CAD build for the part. Positions are in the model's coordinates, mm. A direction names the side the tool comes from. Give positions to 0.01 mm unless a question says otherwise; leave off trailing zeros. Write each loop counter-clockwise with the first axis right and the second up, starting at its lowest first coordinate (ties: lowest second). Pieces come first, ordered by that corner, then holes. Notation, with made-up numbers: (-22, 12.5) - (4, 12.5) arc R22 cw to (4, 48.5) - close; hole circle Ø6 at (47.25, 80). An arc over 180 degrees is marked (long way). Put each result on its own line as item: value. Start each with the question number.
1. Cut at D-D on x = -7.5. List the corners of the cut face in (y, z).
2. Mould opens along X. For faces 1 (the cylindrical face through (16.24, -12.517, 0.76)), 2 (the flat face through (19.5, 0, 1)), 3 (the cylindrical face through (-16.76, 16.483, 0.76)), 4 (the flat face through (-19.5, 0, 1)) say: +X half, -X half, draft (parallel to the pull), parting line (faces both ways), or undercut.
3. Drop flat-ended pins along their axis: pin 1 (2.5 mm diameter, centred on x = -8, z = 7, fed in from +Y); pin 2 (1 mm diameter, centred on y = 0, z = 6, fed in from -X); pin 3 (2 mm diameter, centred on x = 14.5, y = 9.5, fed in from +Z); pin 4 (3.5 mm diameter, centred on x = 16.5, y = -14.5, fed in from -Z) (3 decimals). Give the stop position or say it passes through.
4. Tool access for faces 5 (the flat face through (16.5, 0, 5)), 6 (the flat face through (-3.454, 15, 6)), 7 (the flat face through (-12.5, 15, 6)), 8 (the flat face through (11.5, -14, 5)): list every direction of +Z, -Z, +X, -X, +Y, -Y with a clear straight run to the whole face (end or side of a thin tool).
5. Wall check: line 1 (Y direction, x = 16.5, z = 1.1); line 2 (Y direction, x = -10.5, z = 4.5); line 3 (Y direction, x = -1, z = 7.25). Give the ranges that are in metal, low to high.
6. Cut at B-B on y = -14.5. List the corners of the cut face in (x, z), and give its area (4 significant figures).
7. Cut at A-A on x = -16.5. List the corners of the cut face in (y, z).
8. Cut at C-C on z = 8.25. List the corners of the cut face in (x, y), and give its area (3 significant figures).
from build123d import *

# Parameters (mm, degrees)
ESQUISSE1_W                     = 39
ESQUISSE1_H                     = 35
BOSS_EXTRU_1_DEPTH              = 1.5
ENL_V_MAT_EXTRU_1_REACH         = 28.244
ESQUISSE2_R                     = 2
R_P_TITION_LIN_AIRE1_COUNT      = 2
R_P_TITION_LIN_AIRE1_PITCH      = 33
R_P_TITION_LIN_AIRE1_COUNT_DIR2 = 2
R_P_TITION_LIN_AIRE1_PITCH_DIR2 = 29
ESQUISSE3_W                     = 9.045882094
ESQUISSE3_H                     = 2
BOSS_EXTRU_2_DEPTH              = 9
BOSS_EXTRU_3_DEPTH              = 8


with BuildPart() as part:
    # Esquisse1 → Boss.-Extru.1 (new body)
    with BuildSketch(Plane.XY):
        Rectangle(ESQUISSE1_W, ESQUISSE1_H)
    extrude(amount=BOSS_EXTRU_1_DEPTH)

    # Esquisse2 → Enlèv. mat.-Extru.1 (cut, up to next)
    with BuildSketch(Plane.XY.offset(1.5), mode=Mode.PRIVATE) as enl_v_mat_extru_1_sk1:
        with Locations((16.5, 14.5)):
            Circle(ESQUISSE2_R)
    enl_v_mat_extru_1_tool1 = extrude(enl_v_mat_extru_1_sk1.sketch, amount=-ENL_V_MAT_EXTRU_1_REACH, mode=Mode.PRIVATE) & part.part
    enl_v_mat_extru_1 = enl_v_mat_extru_1_tool1.solids().sort_by_distance((16.5, 14.5, 1.5))[0]
    add(enl_v_mat_extru_1, mode=Mode.SUBTRACT)

    # Répétition linéaire1: Enl_v. mat.-Extru.1 2 × 2
    with Locations(*[(-i * R_P_TITION_LIN_AIRE1_PITCH, -j * R_P_TITION_LIN_AIRE1_PITCH_DIR2, 0) for i in range(R_P_TITION_LIN_AIRE1_COUNT) for j in range(R_P_TITION_LIN_AIRE1_COUNT_DIR2) if (i, j) != (0, 0)]):
        add(enl_v_mat_extru_1, mode=Mode.SUBTRACT)

    # Esquisse3 → Boss.-Extru.2 (add)
    with BuildSketch(Plane.XY.offset(1.5)):
        with Locations((-7.977058953, 15.5)):
            Rectangle(ESQUISSE3_W, ESQUISSE3_H)
    extrude(amount=BOSS_EXTRU_2_DEPTH)

    # Esquisse4 → Boss.-Extru.3 (add)
    with BuildSketch(Plane.XY.offset(1.5)):
        Polygon((-13.5, 10.5), (16.5, 10.5), (16.5, -11.5), (11.5, -11.5), (11.5, -16.5), (-13.5, -16.5), align=None)
    extrude(amount=BOSS_EXTRU_3_DEPTH)


solid = part.part
Report:
1. outline: (-17.5, 0) - (17.5, 0) - (17.5, 1.5) - (16.5, 1.5) - (16.5, 10.5) - (14.5, 10.5) - (14.5, 1.5) - (10.5, 1.5) - (10.5, 9.5) - (-16.5, 9.5) - (-16.5, 1.5) - (-17.5, 1.5) - close
2. face 1: undercut
2. face 2: +X half
2. face 3: undercut
2. face 4: -X half
3. pin 1: stops at y = 16.5
3. pin 2: stops at x = -13.5
3. pin 3: stops at z = 9.5
3. pin 4: passes through
4. face 5: +Z, +X, +Y, -Y
4. face 6: +Z, +X, +Y
4. face 7: +Z, -X, +Y
4. face 8: +Z, +X, -Y
5. line 1: y = -17.5 to -16.5, -12.5 to 12.5, 16.5 to 17.5
5. line 2: y = -16.5 to 10.5, 14.5 to 16.5
5. line 3: y = -16.5 to 10.5
6. outline: (-19.5, 0) - (-18.5, 0) - (-18.5, 1.5) - (-19.5, 1.5) - close; (-14.5, 0) - (14.5, 0) - (14.5, 1.5) - (11.5, 1.5) - (11.5, 9.5) - (-13.5, 9.5) - (-13.5, 1.5) - (-14.5, 1.5) - close; (18.5, 0) - (19.5, 0) - (19.5, 1.5) - (18.5, 1.5) - close
6. area: 246.5 mm²
7. outline: (-17.5, 0) - (-16.5, 0) - (-16.5, 1.5) - (-17.5, 1.5) - close; (-12.5, 0) - (12.5, 0) - (12.5, 1.5) - (-12.5, 1.5) - close; (16.5, 0) - (17.5, 0) - (17.5, 1.5) - (16.5, 1.5) - close
8. outline: (-13.5, -16.5) - (11.5, -16.5) - (11.5, -11.5) - (16.5, -11.5) - (16.5, 10.5) - (-13.5, 10.5) - close; (-12.5, 14.5) - (-3.45, 14.5) - (-3.45, 16.5) - (-12.5, 16.5) - close
8. area: 803 mm²
